Can you work these out from the model? Positions are in its coordinate system, mm. A direction names the side the tool comes from. Give positions to 0.01 mm unless a question says otherwise; leave off trailing zeros. Order: outer loops, then holes, each group sorted by start corner. A loop starts at its lowest first (then second) coordinate and runs counter-clockwise, first axis right, second up. Notation, with made-up numbers: (32.5, 78.25) - (88.5, 78.25) arc R21 cw to (88.5, 106.25) - close; hole circle Ø10 at (-10.5, 33). An arc over 180 degrees is marked (long way). Use one line per item in the form item = value. Start each with the question number.
1) Please list where these lines run through material, in increasing order: probe 1 along Y at (x, z) = (-9, 0.25); probe 2 along Z at (x, y) = (-15, 9.5); probe 3 along X at (y, z) = (8.25, 0).
2) We'd pull the mould along Z, two halves only. Please class faces 1 (the flat face through (3, 1, -5)), 2 (the cylindrical face through (16.265, 4.93, 0.806)), 3 (the flat face through (-3, 8.5, 0)): released by +Z, released by -Z, zero draft, split by the parting line, or undercut.
3) Suppose I cut it at B-B, the plane z = 0. Write out the boundary of the cut face in (x, y).
4) Suppose I cut it at D-D, the plane y = 3. Write out the boundary of the cut face in (x, z).
5) Suppose I cut it at C-C, the plane x = -15. Write out the boundary of the cut face in (y, z), and give its area (3 significant figures).
6) For pin 1 (1.8 mm diameter, centred on x = -15, z = 0, fed in from -Y), with a flat end and sliding along its axis, tell me the tip position at first contact or that it passes through.
7) Which directions (+Z, -Z, +X, -X, +Y, -Y) give clear straight access to the entire face, cutting with the end or side of a thin tool? Please do faces 4 (the cylindrical face through (-14.55, 9.24, 1.43)), 5 (the flat face through (12.5, 5, 0)).
8) Suppose I cut it at A-A, the plane x = 15. Write out the boundary of the cut face in (y, z), and give its area (3 significant figures).
```python
from build123d import *

# Parameters (mm, degrees)
SKETCH1_W           = 35
SKETCH1_H           = 10
SKETCH1_R           = 1.5
BOSS_EXTRUDE1_DEPTH = 10
SKETCH2_W           = 60
SKETCH2_H           = 7
CUT_EXTRUDE1_DEPTH  = 10


with BuildPart() as part:
    # Sketch1 → Boss-Extrude1 (new body)
    with BuildSketch(Plane(origin=(0, 0, 0), x_dir=(1, 0, 0), z_dir=(0, 1, 0))):
        Rectangle(SKETCH1_W, SKETCH1_H)
        with Locations(Location((-15, 0, 0), (0, 0, 270))):
            Circle(SKETCH1_R, mode=Mode.SUBTRACT)
        with Locations(Location((15, 0, 0), (0, 0, 270))):
            Circle(SKETCH1_R, mode=Mode.SUBTRACT)
    extrude(amount=BOSS_EXTRUDE1_DEPTH)

    # Sketch2 → Cut-Extrude1 (cut)
    with BuildSketch(Plane.XY.offset(5)):
        with Locations((-17.5, 5)):
            Rectangle(SKETCH2_W, SKETCH2_H)
    extrude(amount=-CUT_EXTRUDE1_DEPTH, mode=Mode.SUBTRACT)


solid = part.part
```
Result sheet:
q1.probe_1 = 0 to 1.5, 8.5 to 10
q1.probe_2 = -5 to -1.5, 1.5 to 5
q1.probe_3 = 12.5 to 13.5, 16.5 to 17.5
q2.face_1 = released by -Z
q2.face_2 = undercut
q2.face_3 = zero draft
q3.outline = (-17.5, 0) - (-16.5, 0) - (-16.5, 1.5) - (-17.5, 1.5) - close; (-17.5, 8.5) - (-16.5, 8.5) - (-16.5, 10) - (-17.5, 10) - close; (-13.5, 0) - (13.5, 0) - (13.5, 10) - (-13.5, 10) - (-13.5, 8.5) - (12.5, 8.5) - (12.5, 1.5) - (-13.5, 1.5) - close; (16.5, 0) - (17.5, 0) - (17.5, 10) - (16.5, 10) - close
q4.outline = (12.5, -5) - (17.5, -5) - (17.5, 5) - (12.5, 5) - close; hole circle Ø3 at (15, 0)
q5.outline = (0, -5) - (1.5, -5) - (1.5, -1.5) - (0, -1.5) - close; (0, 1.5) - (1.5, 1.5) - (1.5, 5) - (0, 5) - close; (8.5, -5) - (10, -5) - (10, -1.5) - (8.5, -1.5) - close; (8.5, 1.5) - (10, 1.5) - (10, 5) - (8.5, 5) - close
q5.area = 21.0 mm²
q6.pin_1 = through
q7.face_4 = +Y, -Y
q7.face_5 = +Z, -Z, -X
q8.outline = (0, -5) - (10, -5) - (10, -1.5) - (0, -1.5) - close; (0, 1.5) - (10, 1.5) - (10, 5) - (0, 5) - close
q8.area = 70.0 mm²
